The drawing under review shows one solid part. Ordinate dimensions are in mm from its lowest x, y, z. A direction names the side the tool comes from. Round coordinates to 2 decimals unless told otherwise and drop trailing zeros. Write each loop counter-clockwise with the first axis right and the second up, starting at its lowest first coordinate (ties: lowest second). Pieces come first, ordered by that corner, then holes. Notation, with made-up numbers: M 13,-15 L 48,-15 A15 ccw 48,3 Z; hole C -8,68.5 d6. An arc over 180 degrees is marked long. One line per item, written item: value. Start each with the question number.
1) Wall thickness on probe 1 along Y at (x, z) = (6, 2.7); probe 2 along Z at (x, y) = (5.5, 20.5); probe 3 along Y at (x, z) = (4, 5.1): over which ranges is each line inside the solid? List them lowest first.
2) Take a section at C-C, the plane y = 12. Write out the cut boundary in (x, z).
3) Take a section at D-D, the plane x = 6. Write out the cut boundary in (y, z) (1 decimal).
4) Take a section at B-B, the plane z = 2.3. Write out the cut boundary in (x, y).
5) Mouldability with a two-part tool opening along Y and no side actions: class the marked faces 3, 4 and 5 as +Y half, -Y half, draft (parallel to the pull), parting line (faces both ways), or undercut.
6) For P1, Ø6.5, axis at x = 13, y = 40, coming from the +Z side; P2, Ø3, axis at x = 18, z = 5, coming from the +Y side; P3, Ø1, axis at x = 16.5, z = 3, coming from the -Y side; P4, Ø5, axis at x = 9, y = 43.5, coming from the -Z side, all flat-tipped, find the tip position at first contact; note any pin that passes through.
7) Tool access review of the marked faces 1 and 2: name each direction out of +Z, -Z, +X, -X, +Y, -Y from which nothing blocks a thin tool from reaching the whole face with its end or side.
8) Take a section at A-A, the plane x = 13. Write out the cut boundary in (y, z).
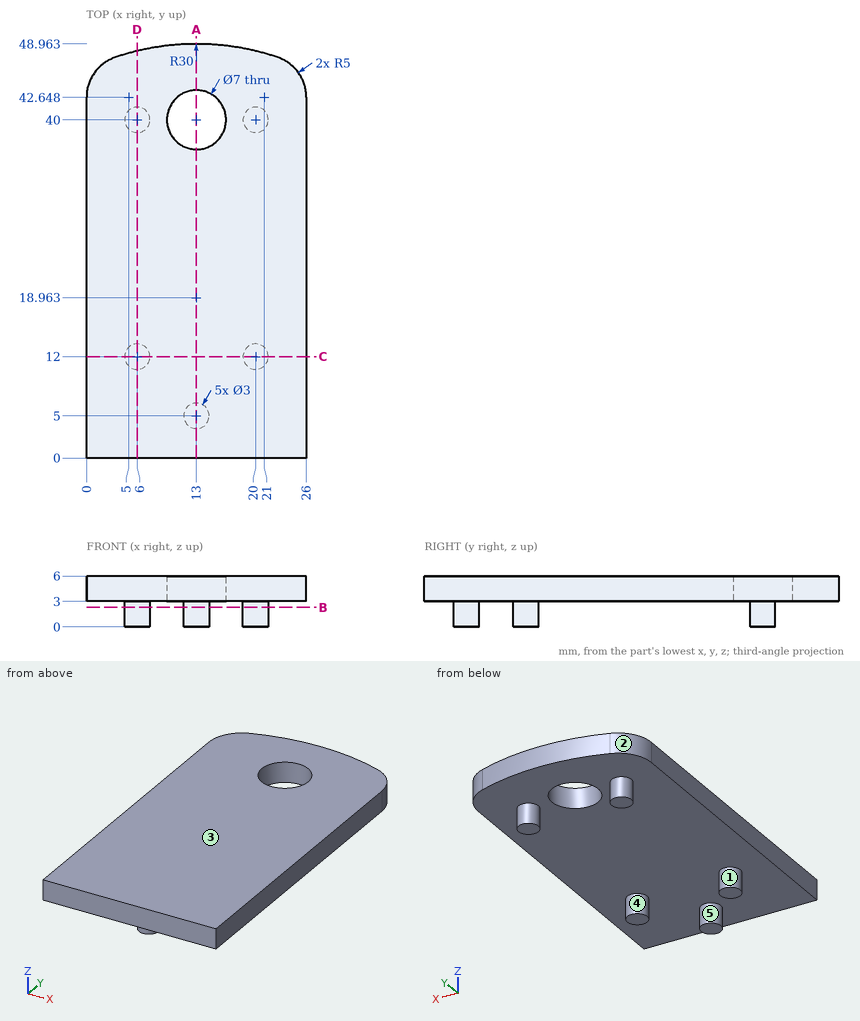
Checked values:
1. probe 1: y = 10.5 to 13.5, 38.5 to 41.5
1. probe 2: z = 3 to 6
1. probe 3: y = 0 to 47.58
2. outline: M 0,3 L 4.5,3 L 4.5,0 L 7.5,0 L 7.5,3 L 18.5,3 L 18.5,0 L 21.5,0 L 21.5,3 L 26,3 L 26,6 L 0,6 Z
3. outline: M 0,3 L 10.5,3 L 10.5,0 L 13.5,0 L 13.5,3 L 38.5,3 L 38.5,0 L 41.5,0 L 41.5,3 L 48.1,3 L 48.1,6 L 0,6 Z
4. outline: C 6,12 d3; C 6,40 d3; C 13,5 d3; C 20,12 d3; C 20,40 d3
5. face 3: draft
5. face 4: undercut
5. face 5: parting line
6. P1: passes through
6. P2: stops at y = 48.76
6. P3: stops at y = 0
6. P4: stops at z = 3
7. face 1: -Z
7. face 2: +Z, -Z, -X, +Y
8. outline: M 0,3 L 3.5,3 L 3.5,0 L 6.5,0 L 6.5,3 L 36.5,3 L 36.5,6 L 0,6 Z; M 43.5,3 L 48.96,3 L 48.96,6 L 43.5,6 Z
